Drawing for the job (mm, zero at the part's lowest x, y, z). Round coordinates to 2 decimals unless told otherwise and drop trailing zeros. Order: outer loops, then holes, each group sorted by start corner. A loop starts at its lowest first (then second) coordinate and runs counter-clockwise, first axis right, second up. Notation, with made-up numbers: M 75,60 L 91,60 A34 ccw 91,90 Z; hole C 38.5,28.5 d3. An arc over 180 degrees is marked long. One line per item, written item: value. Start each with the question number.
Item 1: Probe L1, parallel to Z at x = 12.5, y = 8.75 (1 decimal); L2, parallel to X at y = 3, z = 9; L3, parallel to X at y = 4.5, z = 9. List the from-to ranges inside material, lowest first.
Item 2: Pin check, flat tips, straight feed: pin 1 (1.5 mm diameter, centred on x = 17.5, z = 1, fed in from -Y); pin 2 (1 mm diameter, centred on y = 3.5, z = 4.5, fed in from -X); pin 3 (1.5 mm diameter, centred on x = 28.5, z = 6, fed in from +Y); pin 4 (3 mm diameter, centred on x = 16, z = 7.5, fed in from +Y). Stop position of each tip, or through.
Item 3: Band-saw the part on A-A, the plane z = 5. Write the cut outline in (x, y).
Item 4: Band-saw the part on D-D, the plane x = 5.5. Write the cut outline in (y, z).
Item 5: Band-saw the part on C-C, the plane x = 29. Write the cut outline in (y, z).
Item 6: Two-plate mould, pull along Y, no slides. Class the marked faces 1 and 2: +Y half, -Y half, draft (parallel to the pull), parting line (faces both ways), or undercut.
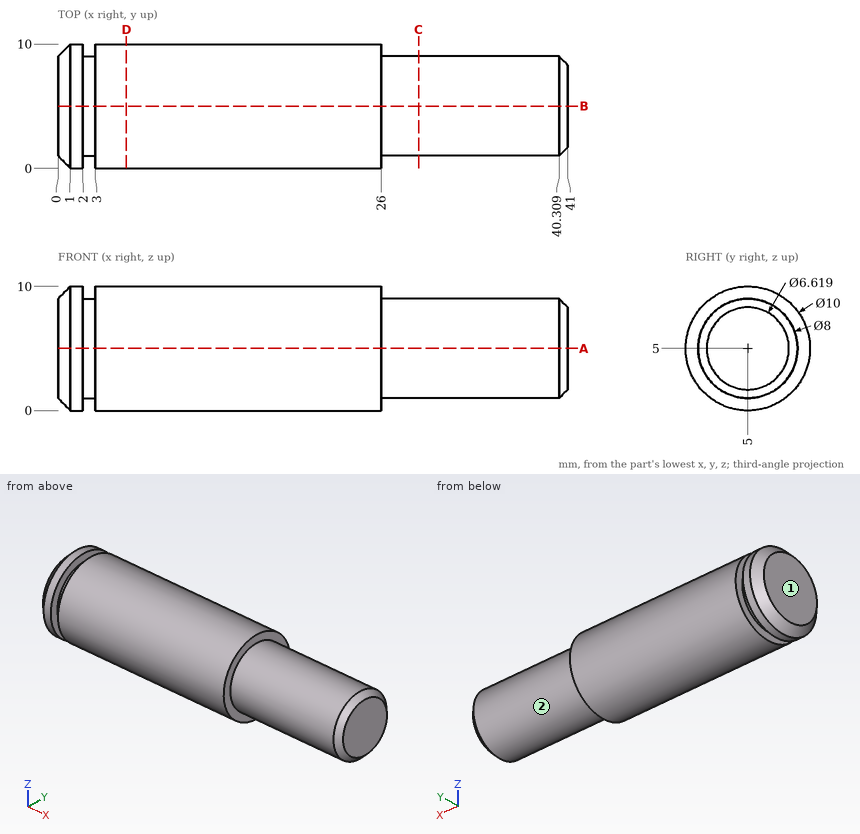
Output:
1. L1: z = 1.7 to 8.3
1. L2: x = 0.47 to 2, 3 to 26
1. L3: x = 0.03 to 2, 3 to 26
2. pin 1: stops at y = 1.2
2. pin 2: stops at x = 0
2. pin 3: stops at y = 8.99
2. pin 4: stops at y = 9.9
3. outline: M 0,1 L 1,0 L 2,0 L 2,1 L 3,1 L 3,0 L 26,0 L 26,1 L 40.31,1 L 41,1.69 L 41,8.31 L 40.31,9 L 26,9 L 26,10 L 3,10 L 3,9 L 2,9 L 2,10 L 1,10 L 0,9 Z
4. outline: C 5,5 d10
5. outline: C 5,5 d8
6. face 1: draft
6. face 2: parting line
